from build123d import *

# Parameters (mm, degrees)
BOSS_EXTRUDE1_DEPTH = 27
SKETCH2_R           = 3.5
CUT_EXTRUDE1_DEPTH  = 8
CUT_EXTRUDE2_DEPTH  = 53.574815946
CUT_EXTRUDE3_REACH  = 151.521
SKETCH5_W           = 1.574815946
SKETCH5_H           = 22
CUT_EXTRUDE4_REACH  = 151.521


with BuildPart() as part:
    # Sketch1 → Boss-Extrude1 (new, symmetric)
    with BuildSketch(Plane.XY):
        Polygon((0, 0), (0, 8), (86.522390311, 8), (97.947574365, 0), (108.271950219, 14.744736797), (152.157870224, -15.984515211), (137.244882879, -37.282468363), (84, 0), align=None)
    extrude(amount=BOSS_EXTRUDE1_DEPTH, both=True)

    # Sketch2 → Cut-Extrude1 (cut)
    with BuildSketch(Plane(origin=(0, 8, 0), x_dir=(1, 0, 0), z_dir=(0, 1, 0))):
        with Locations(Location((11, 16, 0), (0, 0, 180))):
            Circle(SKETCH2_R)
        with Locations(Location((43, 16, 0), (0, 0, 180))):
            Circle(SKETCH2_R)
        with Locations(Location((75, 16, 0), (0, 0, 180))):
            Circle(SKETCH2_R)
        with Locations(Location((11, -16, 0), (0, 0, 180))):
            Circle(SKETCH2_R)
        with Locations(Location((43, -16, 0), (0, 0, 180))):
            Circle(SKETCH2_R)
        with Locations(Location((75, -16, 0), (0, 0, 180))):
            Circle(SKETCH2_R)
    extrude(amount=-CUT_EXTRUDE1_DEPTH, mode=Mode.SUBTRACT)

    # Sketch4 → Cut-Extrude2 (cut)
    with BuildSketch(Plane(origin=(109.609728898, -76.749558436, 0), x_dir=(0, 0, -1), z_dir=(0.8191520442889955, -0.5735764363510408, 0))):
        Polygon((-17.5, 56.180420653), (0, 56.180420653), (0, 74.180420653), (-5, 74.180420653), (-5, 64.180420653), (-17.5, 64.180420653), align=None)
        Polygon((0, 74.180420653), (0, 56.180420653), (17.5, 56.180420653), (17.5, 64.180420653), (5, 64.180420653), (5, 74.180420653), align=None)
    extrude(amount=-CUT_EXTRUDE2_DEPTH, mode=Mode.SUBTRACT)

    # Cut-Extrude3: up to this face of the body (flat: up to its plane)
    cut_extrude3_end = Plane(part.part.faces().sort_by_distance((111.965486474, -9.815447728, 0))[0])
    # Sketch5 → Cut-Extrude3 (cut, up to the picked face)
    with BuildSketch(Plane(origin=(42.548141325, 60.765043225, 0), x_dir=(0.8191520442889958, -0.5735764363510405, 0), z_dir=(0.5735764363510404, 0.8191520442889957, 0)), mode=Mode.PRIVATE) as cut_extrude3_sk1:
        with Locations((81.021363747, 16)):
            Rectangle(SKETCH5_W, SKETCH5_H)
    cut_extrude3_tool1 = split(extrude(cut_extrude3_sk1.sketch, amount=-CUT_EXTRUDE3_REACH, mode=Mode.PRIVATE), bisect_by=cut_extrude3_end, keep=Keep.BOTH, mode=Mode.PRIVATE)
    # Sketch5 → Cut-Extrude3 (cut, up to the picked face)
    with BuildSketch(Plane(origin=(42.548141325, 60.765043225, 0), x_dir=(0.8191520442889958, -0.5735764363510405, 0), z_dir=(0.5735764363510404, 0.8191520442889957, 0)), mode=Mode.PRIVATE) as cut_extrude3_sk2:
        with Locations((81.021363747, -16)):
            Rectangle(SKETCH5_W, SKETCH5_H)
    cut_extrude3_tool2 = split(extrude(cut_extrude3_sk2.sketch, amount=-CUT_EXTRUDE3_REACH, mode=Mode.PRIVATE), bisect_by=cut_extrude3_end, keep=Keep.BOTH, mode=Mode.PRIVATE)
    add(cut_extrude3_tool1.solids().sort_by(Axis((108.916957, 14.293098, -16), (-0.5735764363510404, -0.8191520442889957, 0)))[0], mode=Mode.SUBTRACT)
    add(cut_extrude3_tool2.solids().sort_by(Axis((108.916957, 14.293098, 16), (-0.5735764363510404, -0.8191520442889957, 0)))[0], mode=Mode.SUBTRACT)

    # Cut-Extrude4: up to this face of the body (flat: up to its plane)
    cut_extrude4_end = Plane(part.part.faces().sort_by_distance((110.622441439, -18.641234181, 0))[0])
    # Sketch5<4> → Cut-Extrude4 (cut, up to the picked face)
    with BuildSketch(Plane(origin=(42.548141325, 60.765043225, 0), x_dir=(0.8191520442889958, -0.5735764363510405, 0), z_dir=(0.5735764363510404, 0.8191520442889957, 0)), mode=Mode.PRIVATE) as cut_extrude4_sk1:
        with BuildLine():
            Line((126.249743807, -27), (133.80877172, -27))
            Line((133.80877172, -27), (133.80877172, -17.5))
            Line((133.80877172, -17.5), (133.80877172, -5))
            Line((133.80877172, -5), (133.80877172, 0))
            ThreePointArc((133.80877172, 0), (131.883368816, -14.019084341), (126.249743807, -27))
        make_face()
    cut_extrude4_tool1 = split(extrude(cut_extrude4_sk1.sketch, amount=-CUT_EXTRUDE4_REACH, mode=Mode.PRIVATE), bisect_by=cut_extrude4_end, keep=Keep.BOTH, mode=Mode.PRIVATE)
    # Sketch5<4> → Cut-Extrude4 (cut, up to the picked face)
    with BuildSketch(Plane(origin=(42.548141325, 60.765043225, 0), x_dir=(0.8191520442889958, -0.5735764363510405, 0), z_dir=(0.5735764363510404, 0.8191520442889957, 0)), mode=Mode.PRIVATE) as cut_extrude4_sk2:
        with BuildLine():
            Line((133.567828899, 5), (133.80877172, 5))
            Line((133.80877172, 5), (133.80877172, 17.5))
            Line((133.80877172, 17.5), (133.80877172, 27))
            Line((133.80877172, 27), (126.249743807, 27))
            ThreePointArc((126.249743807, 27), (131.150553282, 16.413061639), (133.567828899, 5))
        make_face()
    cut_extrude4_tool2 = split(extrude(cut_extrude4_sk2.sketch, amount=-CUT_EXTRUDE4_REACH, mode=Mode.PRIVATE), bisect_by=cut_extrude4_end, keep=Keep.BOTH, mode=Mode.PRIVATE)
    # Sketch5<4> → Cut-Extrude4 (cut, up to the picked face)
    with BuildSketch(Plane(origin=(42.548141325, 60.765043225, 0), x_dir=(0.8191520442889958, -0.5735764363510405, 0), z_dir=(0.5735764363510404, 0.8191520442889957, 0)), mode=Mode.PRIVATE) as cut_extrude4_sk3:
        with BuildLine():
            ThreePointArc((133.567828899, 5), (133.748501087, 2.502900989), (133.80877172, 0))
            Line((133.80877172, 0), (133.80877172, 5))
            Line((133.80877172, 5), (133.567828899, 5))
        make_face()
    cut_extrude4_tool3 = split(extrude(cut_extrude4_sk3.sketch, amount=-CUT_EXTRUDE4_REACH, mode=Mode.PRIVATE), bisect_by=cut_extrude4_end, keep=Keep.BOTH, mode=Mode.PRIVATE)
    add(cut_extrude4_tool1.solids().sort_by(Axis((150.325954, -14.701794, 20.352048), (-0.5735764363510404, -0.8191520442889957, 0)))[0], mode=Mode.SUBTRACT)
    add(cut_extrude4_tool2.solids().sort_by(Axis((150.3151, -14.694193, -20.453703), (-0.5735764363510404, -0.8191520442889957, 0)))[0], mode=Mode.SUBTRACT)
    add(cut_extrude4_tool3.solids().sort_by(Axis((152.098683, -15.943072, -3.75058), (-0.5735764363510404, -0.8191520442889957, 0)))[0], mode=Mode.SUBTRACT)


solid = part.part
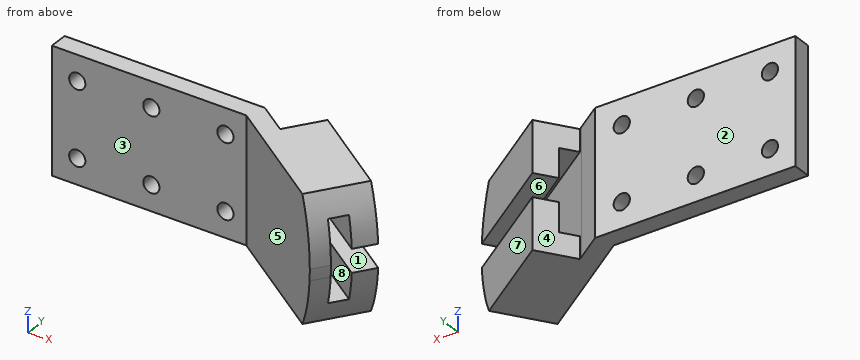
Design review of the part built by this model. Coordinates are the model's own, in mm. Face numbers are marked on the shaded views. A direction names the side the tool comes from. Round coordinates to 2 decimals unless told otherwise and drop trailing zeros. Write each loop counter-clockwise with the first axis right and the second up, starting at its lowest first coordinate (ties: lowest second). Pieces come first, ordered by that corner, then holes.
Item 1: Consider section B-B on y = 4. Count the separate pieces of the cut face and the enclosed holes in it, and give its area (3 significant figures).
Item 2: For pin 1 Ø6.5 at (x, z) = (11, 16) entering from +Y; pin 2 Ø4 at (x, z) = (29.5, -15.5) entering from -Y; pin 3 Ø1 at (x, z) = (43.5, 9) entering from +Y; pin 4 Ø12 at (y, z) = (-19.5, -17.5) entering from +X, all flat-tipped, find the tip position at first contact; note any pin that passes through.
Item 3: Consider section D-D on z = 23. Give the boundary of the cut face in (x, y).
Item 4: Consider section A-A on x = 43. Give the boundary of the cut face in (y, z), and give its area (3 significant figures).
Item 5: For the marked faces 1, 2, 3 and 4, list the 3-axis set-ups (+Z, -Z, +X, -X, +Y, -Y) from which the entire face can be reached by the end or side of a thin tool; tool diameter is ignored.
Item 6: Draft analysis for pull direction X (two halves, no side actions). For the marked faces 5, 6, 7 and 8, state which applies: released by +X, released by -X, zero draft, split by the parting line, or undercut.
Item 7: Consider section C-C on z = 16. Give the boundary of the cut face in (x, y), and give its area (3 significant figures).
Item 8: Wall thickness on L1, parallel to Z at x = 75, y = 2.75; L2, parallel to Y at x = 17.5, z = 14.5; L3, parallel to Y at x = 124, z = 7: over which ranges is each line inside the solid? List them lowest first.
Check values:
1. separate pieces: 3
1. enclosed holes: 6
1. area: 5,580 mm2
2. pin 1: passes through
2. pin 2: stops at y = 0
2. pin 3: stops at y = 8
2. pin 4: stops at x = 150.68
3. outline: (0, 0) - (84, 0) - (132.85, -34.21) - (147.76, -12.91) - (109.56, 13.84) - (99.24, -0.9) - (86.52, 8) - (0, 8) - close
4. outline: (0, -27) - (8, -27) - (8, -19.5) - (0, -19.5) - close; (0, -12.5) - (8, -12.5) - (8, 12.5) - (0, 12.5) - close; (0, 19.5) - (8, 19.5) - (8, 27) - (0, 27) - close
4. area: 320 mm2
5. face 1: +X, +Y
5. face 2: +Z, -Z, -X, +Y
5. face 3: +Z, -Z, -X, -Y
5. face 4: +Z, -Z, +Y
6. face 5: released by -X
6. face 6: zero draft
6. face 7: released by +X
6. face 8: undercut
7. outline: (0, 0) - (7.5, 0) - (7.5, 8) - (0, 8) - close; (14.5, 0) - (39.5, 0) - (39.5, 8) - (14.5, 8) - close; (46.5, 0) - (71.5, 0) - (71.5, 8) - (46.5, 8) - close; (78.5, 0) - (84, 0) - (135.18, -35.84) - (139.77, -29.28) - (86.52, 8) - (78.5, 8) - close; (103.83, 5.65) - (144.36, -22.73) - (150.09, -14.54) - (109.56, 13.84) - close
7. area: 1,520 mm2
8. L1: z = -27 to -19.5, -12.5 to 12.5, 19.5 to 27
8. L2: y = 0 to 8
8. L3: y = -28.01 to -18.24, -8.48 to 3.73
